Input: part model. Units: mm. Frame: model coordinates. Face numbers are marked on the shaded views. A direction names the side the tool comes from. Coordinates: 2 decimals unless noted, no trailing zeros. Loops run counter-clockwise (first coordinate to the right, second up) from the corner with the lowest first, then second, coordinate; pieces in that order, holes last. Notation, with made-up numbers: (-28.75, 5.5) -> (14.25, 5.5) arc R31 ccw to (14.25, 31.5) -> close; hole circle Ø11 at (35, 34). An arc over 180 degrees is marked (long way). Put each result on its own line as item: value. Start each with the question number.
1) Material intervals for L1, parallel to X at y = 0, z = 13; L2, parallel to X at y = 0.1, z = 3.75; L3, parallel to Y at x = -29.65, z = 9, sorted ascending.
2) Cut plane A-A (y = 0). Return the cut outline in (x, z).
3) Cut plane C-C (x = -29.65). Return the cut outline in (y, z), plus the area to 3 significant figures.
4) Cut plane B-B (z = 1.5). Return the cut outline in (x, y), plus the area to 3 significant figures.
5) Set-up query: the marked faces 3 and 4. Return all of +Z, -Z, +X, -X, +Y, -Y with unobstructed straight access to the full face (end or side cutting, diameter ignored); none if empty.
6) Cut plane D-D (z = 8.25). Return the cut outline in (x, y), plus the area to 3 significant figures.
7) Pull-direction query (X, two-part tool) for the marked faces 1 and 2; classes: pulls with the +X half, pulls with the -X half, needs draft (parallel to the pull), parting line crosses it, or undercut.
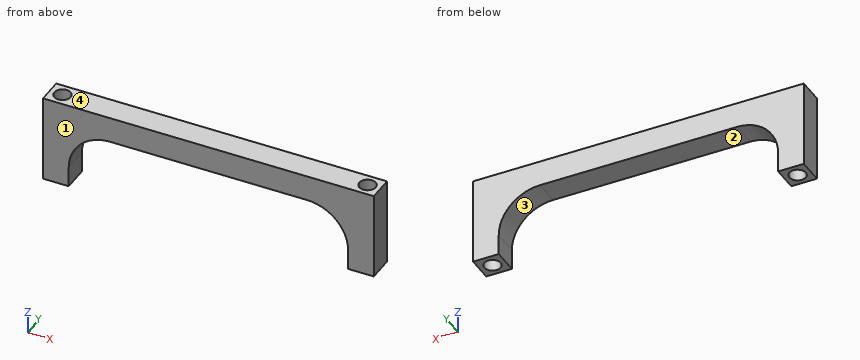
from build123d import *

# Parameters (mm, degrees)
PAD_DEPTH    = 2.5
SKETCH001_R  = 1.6
POCKET_DEPTH = 17.001


with BuildPart() as part:
    # Sketch → Pad (new body, symmetric)
    with BuildSketch(Plane.XZ):
        with BuildLine():
            ThreePointArc((-19.15, 12), (-24.806854, 9.656854), (-27.15, 4))
            Line((-27.15, 0), (-27.15, 4))
            Line((-27.15, 0), (-32.15, 0))
            Line((-32.15, 0), (-32.15, 17))
            Line((-32.15, 17), (32.15, 17))
            Line((32.15, 0), (32.15, 17))
            Line((27.15, 0), (32.15, 0))
            Line((27.15, 0), (27.15, 4))
            ThreePointArc((27.15, 4), (24.806854, 9.656854), (19.15, 12))
            Line((-19.15, 12), (19.15, 12))
        make_face()
    extrude(amount=PAD_DEPTH, both=True)

    # Sketch001 → Pocket (cut, through all)
    with BuildSketch(Plane.XY):
        with Locations((-29.65, 0)):
            Circle(SKETCH001_R)
        with Locations((29.65, 0)):
            Circle(SKETCH001_R)
    extrude(amount=POCKET_DEPTH, mode=Mode.SUBTRACT)


solid = part.part
Results found:
1. L1: x = -32.15 to -31.25, -28.05 to 28.05, 31.25 to 32.15
1. L2: x = -32.15 to -31.25, -28.05 to -27.15, 27.15 to 28.05, 31.25 to 32.15
1. L3: y = -2.5 to -1.6, 1.6 to 2.5
2. outline: (-32.15, 0) -> (-31.25, 0) -> (-31.25, 17) -> (-32.15, 17) -> close; (-28.05, 0) -> (-27.15, 0) -> (-27.15, 4) arc R8 cw to (-19.15, 12) -> (19.15, 12) arc R8 cw to (27.15, 4) -> (27.15, 0) -> (28.05, 0) -> (28.05, 17) -> (-28.05, 17) -> close; (31.25, 0) -> (32.15, 0) -> (32.15, 17) -> (31.25, 17) -> close
3. outline: (-2.5, 0) -> (-1.6, 0) -> (-1.6, 17) -> (-2.5, 17) -> close; (1.6, 0) -> (2.5, 0) -> (2.5, 17) -> (1.6, 17) -> close
3. area: 30.6 mm2
4. outline: (-32.15, -2.5) -> (-27.15, -2.5) -> (-27.15, 2.5) -> (-32.15, 2.5) -> close; (27.15, -2.5) -> (32.15, -2.5) -> (32.15, 2.5) -> (27.15, 2.5) -> close; hole circle Ø3.2 at (-29.65, 0); hole circle Ø3.2 at (29.65, 0)
4. area: 33.9 mm2
5. face 3: -Z, +Y, -Y
5. face 4: +Z, +X, -X, +Y, -Y
6. outline: (-32.15, -2.5) -> (-25.93, -2.5) -> (-25.93, 2.5) -> (-32.15, 2.5) -> close; (25.93, -2.5) -> (32.15, -2.5) -> (32.15, 2.5) -> (25.93, 2.5) -> close; hole circle Ø3.2 at (-29.65, 0); hole circle Ø3.2 at (29.65, 0)
6. area: 46.1 mm2
7. face 1: needs draft
7. face 2: undercut
